Check sheet for the modelled part. Datum: model origin and axes. Units: mm. A direction names the side the tool comes from. Coordinates: 2 decimals unless noted, no trailing zeros. Loops run counter-clockwise (first coordinate to the right, second up) from the corner with the lowest first, then second, coordinate; pieces in that order, holes last. Notation, with made-up numbers: M -1.5,82.5 L 24.5,82.5 A16 cw 24.5,105.5 Z; hole C -25,-36 d9. An arc over 180 degrees is marked long. Write each question's results on one line, items separated by ' | '. Start each with the question number.
from build123d import *

# Parameters (mm, degrees)
EXTRUDE_1_DEPTH     = 5
EXTRUDE_5_DEPTH     = 5
CUT_EXTRUDE_2_REACH = 82.139
SKETCH_7_R          = 7.5
SKETCH_8_R          = 8.75
CUT_EXTRUDE_3_DEPTH = 1.3
CUT_EXTRUDE_4_REACH = 82.139
SKETCH_9_R          = 1.35
CUT_EXTRUDE_5_REACH = 82.139
SKETCH_12_R         = 2.1
SKETCH_14_W         = 40
SKETCH_14_H         = 7
EXTRUDE_6_DEPTH     = 15
CHAMFER_1_SIZE      = 7
CHAMFER_1_SIZE2     = 3
CUT_EXTRUDE_6_REACH = 134.447
SKETCH_15_R         = 2
FILLET_3_R          = 2
CHAMFER_2_SIZE      = 5
CUT_EXTRUDE_7_DEPTH = 15
SKETCH_17_R         = 7.5
SKETCH_17_R_2       = 2.1
EXTRUDE_7_DEPTH     = 2
CHAMFER_3_SIZE      = 2


# Some blends are built 0.0001 mm under size
with BuildPart() as part:
    # 草图1 → 凸台-拉伸1 (new body)
    with BuildSketch(Plane(origin=(0, 0, 0), x_dir=(1, 0, 0), z_dir=(0, 1, 0))):
        with BuildLine():
            Line((-65, 12.5), (65, 12.5))
            ThreePointArc((65, 12.5), (77.5, 0), (65, -12.5))
            Line((65, -12.5), (-65, -12.5))
            ThreePointArc((-65, -12.5), (-77.5, 0), (-65, 12.5))
        make_face()
    extrude(amount=EXTRUDE_1_DEPTH)

    # 草图10 → 凸台-拉伸5 (add)
    with BuildSketch(Plane.XZ):
        with BuildLine():
            Line((75.795454545, -6.301441197), (78.590909091, -1.512345887))
            ThreePointArc((78.590909091, -1.512345887), (79, 0), (78.590909091, 1.512345887))
            Line((78.590909091, 1.512345887), (75.795454545, 6.301441197))
            Line((75.795454545, 6.301441197), (75.795454545, -6.301441197))
        make_face()
    extrude(amount=-EXTRUDE_5_DEPTH)

    # 草图7 → 切除-拉伸2 (cut, up to next)
    with BuildSketch(Plane(origin=(0, 5, 0), x_dir=(1, 0, 0), z_dir=(0, 1, 0)), mode=Mode.PRIVATE) as cut_extrude_2_sk1:
        with Locations(Location((65, 0, 0), (0, 0, 270))):
            Circle(SKETCH_7_R)
    cut_extrude_2_tool1 = extrude(cut_extrude_2_sk1.sketch, amount=-CUT_EXTRUDE_2_REACH, mode=Mode.PRIVATE) & part.part
    add(cut_extrude_2_tool1.solids().sort_by_distance((65, 5, 0))[0], mode=Mode.SUBTRACT)

    # 草图8 → 切除-拉伸3 (cut)
    with BuildSketch(Plane(origin=(0, 0, 0), x_dir=(1, 0, 0), z_dir=(0, 1, 0))):
        with Locations(Location((65, 0, 0), (0, 0, 270))):
            Circle(SKETCH_8_R)
    extrude(amount=CUT_EXTRUDE_3_DEPTH, mode=Mode.SUBTRACT)

    # 草图9 → 切除-拉伸4 (cut, up to next)
    with BuildSketch(Plane.XZ, mode=Mode.PRIVATE) as cut_extrude_4_sk1:
        with Locations(Location((59.625, 9.309773091, 0), (0, 0, 270))):
            Circle(SKETCH_9_R)
    cut_extrude_4_tool1 = extrude(cut_extrude_4_sk1.sketch, amount=-CUT_EXTRUDE_4_REACH, mode=Mode.PRIVATE) & part.part
    # 草图9 → 切除-拉伸4 (cut, up to next)
    with BuildSketch(Plane.XZ, mode=Mode.PRIVATE) as cut_extrude_4_sk2:
        with Locations(Location((75.75, 0, 0), (0, 0, 270))):
            Circle(SKETCH_9_R)
    cut_extrude_4_tool2 = extrude(cut_extrude_4_sk2.sketch, amount=-CUT_EXTRUDE_4_REACH, mode=Mode.PRIVATE) & part.part
    # 草图9 → 切除-拉伸4 (cut, up to next)
    with BuildSketch(Plane.XZ, mode=Mode.PRIVATE) as cut_extrude_4_sk3:
        with Locations(Location((59.625, -9.309773091, 0), (0, 0, 270))):
            Circle(SKETCH_9_R)
    cut_extrude_4_tool3 = extrude(cut_extrude_4_sk3.sketch, amount=-CUT_EXTRUDE_4_REACH, mode=Mode.PRIVATE) & part.part
    add(cut_extrude_4_tool1.solids().sort_by_distance((59.625, 0, 9.309773))[0], mode=Mode.SUBTRACT)
    add(cut_extrude_4_tool2.solids().sort_by_distance((75.75, 0, 0))[0], mode=Mode.SUBTRACT)
    add(cut_extrude_4_tool3.solids().sort_by_distance((59.625, 0, -9.309773))[0], mode=Mode.SUBTRACT)

    # 草图12 → 切除-拉伸5 (cut, up to next)
    with BuildSketch(Plane(origin=(0, 5, 0), x_dir=(1, 0, 0), z_dir=(0, 1, 0)), mode=Mode.PRIVATE) as cut_extrude_5_sk1:
        with Locations(Location((-65, 0, 0), (0, 0, 270))):
            Circle(SKETCH_12_R)
    cut_extrude_5_tool1 = extrude(cut_extrude_5_sk1.sketch, amount=-CUT_EXTRUDE_5_REACH, mode=Mode.PRIVATE) & part.part
    add(cut_extrude_5_tool1.solids().sort_by_distance((-65, 5, 0))[0], mode=Mode.SUBTRACT)

    # 草图14 → 凸台-拉伸6 (add)
    with BuildSketch(Plane.XZ):
        with Locations((-32, -9)):
            Rectangle(SKETCH_14_W, SKETCH_14_H)
    extrude(amount=EXTRUDE_6_DEPTH)

    # 倒角1
    chamfer_1_edges = [part.edges().sort_by_distance(p)[0] for p in [
        (-52, -7.5, -5.5),
    ]]
    chamfer_1_side = [part.faces().sort_by_distance(p)[0] for p in [
        (-32, -7.5, -5.5),
    ]]
    chamfer(chamfer_1_edges, length=CHAMFER_1_SIZE, length2=CHAMFER_1_SIZE2, reference=chamfer_1_side[0])

    # 草图15 → 切除-拉伸6 (cut, up to next)
    with BuildSketch(Plane.ZY.offset(52), mode=Mode.PRIVATE) as cut_extrude_6_sk1:
        with Locations((-4.5, -12.5)):
            Circle(SKETCH_15_R)
    cut_extrude_6_tool1 = extrude(cut_extrude_6_sk1.sketch, amount=-CUT_EXTRUDE_6_REACH, mode=Mode.PRIVATE) & part.part
    add(cut_extrude_6_tool1.solids().sort_by_distance((-52, -12.5, -4.5))[0], mode=Mode.SUBTRACT)

    # 圆角3
    # the kernel refuses this fillet: 2 mm, written as the material it takes off along each edge
    with BuildSketch(Plane(origin=(-52, 0, -8.5), x_dir=(0.9191450300180579, 0, 0.39391929857916774), z_dir=(0, -1, 0))) as fillet_3_piece_1:
        with BuildLine():
            CenterArc((FILLET_3_R * 0.659396157981, -FILLET_3_R), FILLET_3_R, 90, 66.801409486)
            Line((-FILLET_3_R * 0.259748872037, -FILLET_3_R * 0.606080701421), (0, 0))
            Line((0, 0), (FILLET_3_R * 0.659396157981, 0))
        make_face()
    extrude(amount=18.29698079, mode=Mode.SUBTRACT)
    with BuildSketch(Plane(origin=(-52, 0, -12.5), x_dir=(0, 0, 1), z_dir=(0, -1, 0))) as fillet_3_piece_2:
        with BuildLine():
            CenterArc((FILLET_3_R, -FILLET_3_R), FILLET_3_R, 90, 90)
            Line((0, -FILLET_3_R), (0, 0))
            Line((0, 0), (FILLET_3_R, 0))
        make_face()
    extrude(amount=20, mode=Mode.SUBTRACT)
    with BuildSketch(Plane(origin=(-45, -13.205762298, -5.5), x_dir=(-0.9191450300180575, 0, -0.3939192985791687), z_dir=(0, -1, 0))) as fillet_3_piece_3:
        with BuildLine():
            CenterArc((FILLET_3_R * 0.205257701955, FILLET_3_R), FILLET_3_R, 246.801409486, 23.198590514)
            Line((-FILLET_3_R * 0.188661596625, FILLET_3_R * 0.0808549699819), (0, 0))
            Line((0, 0), (FILLET_3_R * 0.205257701955, 0))
        make_face()
    extrude(amount=2.820526212, mode=Mode.SUBTRACT)
    with BuildSketch(Plane(origin=(-45, 0, -5.5), x_dir=(1, 0, 0), z_dir=(0, -1, 0))) as fillet_3_piece_4:
        with BuildLine():
            CenterArc((FILLET_3_R * 0.205257701955, -FILLET_3_R), FILLET_3_R, 90, 23.198590514)
            Line((-FILLET_3_R * 0.188661596625, -FILLET_3_R * 0.0808549699819), (0, 0))
            Line((0, 0), (FILLET_3_R * 0.205257701955, 0))
        make_face()
    extrude(amount=11.794237702, mode=Mode.SUBTRACT)
    with BuildSketch(Plane(origin=(-12, 0, -5.5), x_dir=(-1, 0, 0), z_dir=(0, -1, 0))) as fillet_3_piece_5:
        with BuildLine():
            CenterArc((FILLET_3_R, FILLET_3_R), FILLET_3_R, 180, 90)
            Line((0, FILLET_3_R), (0, 0))
            Line((0, 0), (FILLET_3_R, 0))
        make_face()
    extrude(amount=15.767949192, mode=Mode.SUBTRACT)
    with BuildSketch(Plane(origin=(-12, -9.232050808, -5.5), x_dir=(0, 0, -1), z_dir=(0, -1, 0))) as fillet_3_piece_6:
        with BuildLine():
            CenterArc((FILLET_3_R, -FILLET_3_R), FILLET_3_R, 90, 90)
            Line((0, -FILLET_3_R), (0, 0))
            Line((0, 0), (FILLET_3_R, 0))
        make_face()
    extrude(amount=10.767949192, mode=Mode.SUBTRACT)
    with BuildSketch(Plane(origin=(-12, 0, -12.5), x_dir=(0, 0, 1), z_dir=(0, -1, 0))) as fillet_3_piece_7:
        with BuildLine():
            CenterArc((FILLET_3_R, FILLET_3_R), FILLET_3_R, 180, 90)
            Line((0, FILLET_3_R), (0, 0))
            Line((0, 0), (FILLET_3_R, 0))
        make_face()
    extrude(amount=20, mode=Mode.SUBTRACT)

    # 倒角2
    chamfer_2_edges = [part.edges().sort_by_distance(p)[0] for p in [
        (-29.294742298, 0, -5.5),
        (-12, 0, -9),
        (-51.669682184, 0, -8.717810298),
        (-51.414213562, 0, -11.914213562),
        (-44.991616341, 0, -5.540844554),
        (-12.585786438, 0, -6.085786438),
        (-12.585786438, 0, -11.914213562),
        (-52, 0, -10.159396158),
        (-48.082580895, 0, -6.821106098),
    ]]
    chamfer(chamfer_2_edges, length=CHAMFER_2_SIZE)

    # 草图16 → 切除-拉伸7 (cut)
    with BuildSketch(Plane.XZ.offset(15)):
        Polygon((-61.333333333, -12.5), (-33.333333333, -0.5), (-61.333333333, -0.5), align=None)
    extrude(amount=-CUT_EXTRUDE_7_DEPTH, mode=Mode.SUBTRACT)

    # 草图17 → 凸台-拉伸7 (add)
    with BuildSketch(Plane.XZ):
        with Locations(Location((-65, 0, 0), (0, 0, 90))):
            Circle(SKETCH_17_R)
        with Locations(Location((-65, 0, 0), (0, 0, 90))):
            Circle(SKETCH_17_R_2, mode=Mode.SUBTRACT)
    extrude(amount=EXTRUDE_7_DEPTH)

    # 倒角3
    chamfer_3_edges = [part.edges().sort_by_distance(p)[0] for p in [
        (-65, -2, -7.5),
    ]]
    chamfer(chamfer_3_edges, length=CHAMFER_3_SIZE - 0.0001)  # a hair under: the kernel refuses the full size


solid = part.part
1) Section check A-A (x = 8). Enter the section's corners in (y, z), then the cut area to 3 significant figures.
2) Gauge pin test, flat ends, axial feed: P1, Ø4.5, axis at x = 59.62, z = -9.31, coming from the -Y side; P2, Ø6, axis at y = 3, z = -8, coming from the -X side; P3, Ø0.5, axis at y = -7.5, z = -10.5, coming from the -X side. Record the tip position at first contact, or that the pin passes through.
3) Release check for a two-part mould opening along X. For faces 1 (the cylindrical face through (73.676, 0.641, -1.139)), 2 (the cylindrical face through (-30.2, -12.5, -6.5)), 3 (the flat face through (77.213, 2.465, 3.873)) record: +X half, -X half, draft (parallel to the pull), parting line (faces both ways), or undercut.
4) Set-up check for faces 4 (the flat face through (-12, -10, -9)), 5 (the flat face through (-26.1, -2.5, -3)), 6 (the flat face through (72, 1.3, -4)), 7 (the flat face through (-30, -8, -5.5)): record each of +Z, -Z, +X, -X, +Y, -Y from which the full face is reachable in a straight line by a thin tool's end or side.
5) Thickness scan on probe 1 along Y at (x, z) = (50.5, -6.75); probe 2 along Z at (x, y) = (-22, -9.75); probe 3 along Z at (x, y) = (-65, 3.5). Record the ranges inside material, lowest first.
Return value:
1) outline: M 0,-12.5 L 5,-12.5 L 5,12.5 L 0,12.5 Z | area: 125 mm2
2) P1: stops at y = 0 | P2: stops at x = -76.46 | P3: stops at x = -52
3) face 1: undercut | face 2: draft | face 3: +X half
4) face 4: +Z, -Z, +X, -Y | face 5: +Z, +X, -Y | face 6: -Y | face 7: +Z, +X, -X, -Y
5) probe 1: y = 0 to 5 | probe 2: z = -12.5 to -5.5 | probe 3: z = -12.5 to -2.1, 2.1 to 12.5
